```python
from build123d import *

# Parameters (mm, degrees)
SKETCH_1_W          = 30
SKETCH_1_H          = 30
EXTRUDE_1_DEPTH     = 250
SKETCH_2_W          = 26
SKETCH_2_H          = 26
CUT_EXTRUDE_1_DEPTH = 254.574446662
SKETCH_3_R          = 6
CUT_EXTRUDE_2_DEPTH = 254.574446662
SKETCH_6_R          = 6
CUT_EXTRUDE_4_DEPTH = 254.574446662
CUT_EXTRUDE_5_DEPTH = 254.574446662
CUT_EXTRUDE_6_DEPTH = 254.574446662


with BuildPart() as part:
    # Эскиз1 → Бобышка-Вытянуть1 (new body)
    with BuildSketch(Plane(origin=(0, 0, 0), x_dir=(1, 0, 0), z_dir=(0, 1, 0))):
        with Locations((15, 15)):
            Rectangle(SKETCH_1_W, SKETCH_1_H)
    extrude(amount=EXTRUDE_1_DEPTH)

    # Эскиз2 → Вырез-Вытянуть1 (cut, through all)
    with BuildSketch(Plane(origin=(0, 250, 0), x_dir=(1, 0, 0), z_dir=(0, 1, 0))):
        with Locations((15, 15)):
            Rectangle(SKETCH_2_W, SKETCH_2_H)
    extrude(amount=-CUT_EXTRUDE_1_DEPTH, mode=Mode.SUBTRACT)

    # Эскиз3 → Вырез-Вытянуть2 (cut, through all)
    with BuildSketch(Plane.XY):
        with Locations((15, 15)):
            Circle(SKETCH_3_R)
    extrude(amount=-CUT_EXTRUDE_2_DEPTH, mode=Mode.SUBTRACT)

    # Эскиз6 → Вырез-Вытянуть4 (cut, through all)
    with BuildSketch(Plane.XY):
        with Locations((15, 237)):
            Circle(SKETCH_6_R)
    extrude(amount=-CUT_EXTRUDE_4_DEPTH, mode=Mode.SUBTRACT)

    # Эскиз8 → Вырез-Вытянуть5 (cut, through all)
    with BuildSketch(Plane.XY):
        Polygon((15, 250), (30, 235), (30, 250), align=None)
    extrude(amount=-CUT_EXTRUDE_5_DEPTH, mode=Mode.SUBTRACT)

    # Эскиз9 → Вырез-Вытянуть6 (cut, through all)
    with BuildSketch(Plane.XY):
        Polygon((15, 0), (0, 15), (0, 0), align=None)
    extrude(amount=-CUT_EXTRUDE_6_DEPTH, mode=Mode.SUBTRACT)


solid = part.part
```
The listing builds one solid part. Answer for the finished solid, in the listing's coordinates (mm). A direction names the side the tool comes from. Give positions to 0.01 mm unless a question says otherwise; leave off trailing zeros. Order: outer loops, then holes, each group sorted by start corner. A loop starts at its lowest first (then second) coordinate and runs counter-clockwise, first axis right, second up. Notation, with made-up numbers: (37, -1.75) -> (53, -1.75) arc R18 cw to (53, 33.25) -> close; hole circle Ø2 at (1.5, -26.5). An arc over 180 degrees is marked (long way). Answer as a JSON object with one key per item and string values. Group by question number.
Item 1: The part is cut by section C-C on y = 219. Write down the section's boundary in (x, z), and give its area (3 significant figures).
Item 2: The part is cut by section B-B on x = 23.25. Write down the section's boundary in (y, z).
Item 3: A tool of negligible diameter and unlimited length cuts with its end or side. For faces 1 (the flat face through (29, 0, -14)), 2 (the flat face through (15, 127, -2)), from which of +Z, -Z, +X, -X, +Y, -Y can it reach the whole face along a straight path? Write none if from no direction.
Item 4: The part is cut by section A-A on z = -6. Write down the section's boundary in (x, y).
Item 5: Determine the mould class of faces 3 (the flat face through (28, 120, -15)), 4 (the flat face through (30, 116, -15)), 5 (the flat face through (15, 123, -30)) for opening direction X: pulls with the +X half, pulls with the -X half, needs draft (parallel to the pull), parting line crosses it, or undercut.
Item 6: The part is cut by section D-D on x = 11.25. Write down the section's boundary in (y, z).
Item 7: Consider L1, parallel to Y at x = 15, z = -28.7; L2, parallel to X at y = 45.5, z = -13.5; L3, parallel to Z at x = 25.5, y = 179. Determine where each line is inside the solid, lowest interval first. Write a range as from..to.
Result set:
{
 "1": {"outline": "(0, -30) -> (30, -30) -> (30, 0) -> (0, 0) -> close; hole (2, -28) -> (28, -28) -> (28, -2) -> (2, -2) -> close", "area": "224 mm²"},
 "2": {"outline": "(0, -30) -> (241.75, -30) -> (241.75, -28) -> (0, -28) -> close; (0, -2) -> (241.75, -2) -> (241.75, 0) -> (0, 0) -> close"},
 "3": {"face 1": "+Z, -Z, +X, -X, -Y", "face 2": "+Y, -Y"},
 "4": {"outline": "(0, 15) -> (2, 13) -> (2, 250) -> (0, 250) -> close; (28, 0) -> (30, 0) -> (30, 235) -> (28, 237) -> close"},
 "5": {"face 3": "undercut", "face 4": "pulls with the +X half", "face 5": "needs draft"},
 "6": {"outline": "(3.75, -30) -> (10.32, -30) -> (10.32, -28) -> (3.75, -28) -> close; (3.75, -2) -> (10.32, -2) -> (10.32, 0) -> (3.75, 0) -> close; (19.68, -30) -> (232.32, -30) -> (232.32, -28) -> (19.68, -28) -> close; (19.68, -2) -> (232.32, -2) -> (232.32, 0) -> (19.68, 0) -> close; (241.68, -30) -> (250, -30) -> (250, -28) -> (241.68, -28) -> close; (241.68, -2) -> (250, -2) -> (250, 0) -> (241.68, 0) -> close"},
 "7": {"L1": "0..9, 21..231, 243..250", "L2": "0..2, 28..30", "L3": "-30..-28, -2..0"}
}
